Input: part model. Units: mm. Frame: model coordinates. Face numbers are marked on the shaded views. A direction names the side the tool comes from. Give positions to 0.01 mm unless a question says otherwise; leave off trailing zeros. Loops run counter-clockwise (first coordinate to the right, second up) from the corner with the lowest first, then second, coordinate; pieces in that order, holes last. Notation, with made-up numbers: M -2.75,-39.75 L 16.25,-39.75 A34 ccw 16.25,-4.75 Z; hole C 66.25,-32 d9. An arc over 180 degrees is marked long. Return JSON: item names as keys, results as strings. Group by question number.
```python
from build123d import *

# Parameters (mm, degrees)
SKETCH1_R           = 12
BOSS_EXTRUDE1_DEPTH = 47.625
CUT_EXTRUDE1_START  = -36
SKETCH2_W           = 72
SKETCH2_H           = 38.1
CUT_EXTRUDE1_DEPTH  = 124.587407476
SKETCH3_R           = 36
BOSS_EXTRUDE2_DEPTH = 16
SKETCH4_R           = 15
CUT_EXTRUDE2_DEPTH  = 175.528337599


with BuildPart() as part:
    # Sketch1 → Boss-Extrude1 (new, symmetric)
    with BuildSketch(Plane(origin=(0, 0, 0), x_dir=(1, 0, 0), z_dir=(0, 1, 0))):
        with BuildLine():
            Line((0, -36), (0, 36))
            Line((0, 36), (-112, 36))
            ThreePointArc((-112, 36), (-148, 0), (-112, -36))
            Line((-112, -36), (0, -36))
        make_face()
        with Locations(Location((-112, 0, 0), (0, 0, 270))):
            Circle(SKETCH1_R, mode=Mode.SUBTRACT)
    extrude(amount=BOSS_EXTRUDE1_DEPTH, both=True)

    # Sketch2 → Cut-Extrude1 (cut, through all)
    with BuildSketch(Plane(origin=(0, 0, 0), x_dir=(0, 0, -1), z_dir=(1, 0, 0)).offset(CUT_EXTRUDE1_START)):
        Rectangle(SKETCH2_W, SKETCH2_H)
    extrude(amount=-CUT_EXTRUDE1_DEPTH, mode=Mode.SUBTRACT)

    # Sketch3 → Boss-Extrude2 (add)
    with BuildSketch(Plane(origin=(0, 0, 0), x_dir=(0, 0, -1), z_dir=(1, 0, 0))):
        Circle(SKETCH3_R)
    extrude(amount=BOSS_EXTRUDE2_DEPTH)

    # Sketch4 → Cut-Extrude2 (cut, through all)
    with BuildSketch(Plane(origin=(16, 0, 0), x_dir=(0, 0, -1), z_dir=(1, 0, 0))):
        Circle(SKETCH4_R)
    extrude(amount=-CUT_EXTRUDE2_DEPTH, mode=Mode.SUBTRACT)


solid = part.part
```
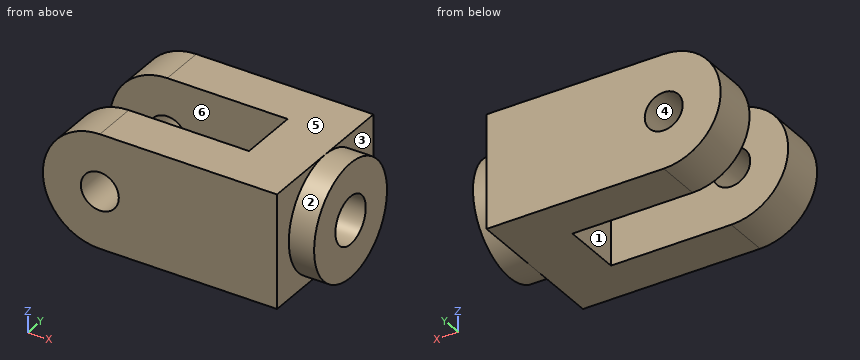
Item 1: Material intervals for line 1 (Y direction, x = -58.5, z = -24.5) (3 decimals); line 2 (X direction, y = 37, z = 0); line 3 (Y direction, x = -16, z = 0) (3 decimals), sorted ascending. Write a range as from..to.
Item 2: Reachability of the marked faces 1, 2 and 3 from +Z, -Z, +X, -X, +Y, -Y: full face, straight path, thin tool, end or side. Return the list, or none.
Item 3: Pull-direction query (Z, two-part tool) for the marked faces 4, 5 and 6; classes: pulls with the +Z half, pulls with the -Z half, needs draft (parallel to the pull), parting line crosses it, or undercut.
Item 4: Section D-D, the plane y = 5.5. Return loops of the section in (x, z).
Item 5: Section A-A, the plane z = 0. Return loops of the section in (x, y) (3 decimals).
Item 6: Section C-C, the plane x = -14. Return loops of the section in (y, z) (3 decimals).
Item 7: Section B-B, the plane y = -40. Return loops of the section in (x, z), then the cut area to 3 significant figures.
Answer below:
{
 "1": {"line 1": "-47.625..-19.05, 19.05..47.625", "line 2": "-148..-124, -100..0", "line 3": "-47.625..-15, 15..47.625"},
 "2": {"face 1": "+Z, -Z, -X", "face 2": "+X", "face 3": "+X, +Y"},
 "3": {"face 4": "undercut", "face 5": "pulls with the +Z half", "face 6": "needs draft"},
 "4": {"outline": "M -36,-36 L 0,-36 L 0,-35.58 L 16,-35.58 L 16,-13.96 L -36,-13.96 Z; M -36,13.96 L 16,13.96 L 16,35.58 L 0,35.58 L 0,36 L -36,36 Z"},
 "5": {"outline": "M -148,-47.625 L -124,-47.625 L -124,-19.05 L -148,-19.05 Z; M -148,19.05 L -124,19.05 L -124,47.625 L -148,47.625 Z; M -100,-47.625 L 0,-47.625 L 0,-36 L 16,-36 L 16,-15 L -36,-15 L -36,-19.05 L -100,-19.05 Z; M -100,19.05 L -36,19.05 L -36,15 L 16,15 L 16,36 L 0,36 L 0,47.625 L -100,47.625 Z"},
 "6": {"outline": "M -47.625,-36 L 47.625,-36 L 47.625,36 L -47.625,36 Z; hole C 0,0 d30"},
 "7": {"outline": "M -112,-36 L 0,-36 L 0,36 L -112,36 A36 ccw Z; hole C -112,0 d24", "area": "9,650 mm^2"}
}
